from build123d import *

# Parameters (mm, degrees)
SKETCH1_W           = 7.874
SKETCH1_H           = 14.0081
BOSS_EXTRUDE1_DEPTH = 2.54
SKETCH2_W           = 1.101725
SKETCH2_H           = 1.0033
CUT_EXTRUDE1_DEPTH  = 8.636
BOSS_EXTRUDE3_DEPTH = 0.7239


with BuildPart() as part:
    # Sketch1 → Boss-Extrude1 (new body)
    with BuildSketch(Plane(origin=(0, 0, 0), x_dir=(1, 0, 0), z_dir=(0, 1, 0))):
        with Locations((3.937, 7.00405)):
            Rectangle(SKETCH1_W, SKETCH1_H)
    extrude(amount=BOSS_EXTRUDE1_DEPTH)

    # Sketch2 → Cut-Extrude1 (cut)
    with BuildSketch(Plane(origin=(0, 0, -14.0081), x_dir=(-1, 0, 0), z_dir=(0, 0, -1))):
        with Locations((-6.4976375, 1.36525)):
            Rectangle(SKETCH2_W, SKETCH2_H)
        with Locations((-3.971925, 1.36525)):
            Rectangle(SKETCH2_W, SKETCH2_H)
        with Locations((-1.4462125, 1.36525)):
            Rectangle(SKETCH2_W, SKETCH2_H)
    extrude(amount=-CUT_EXTRUDE1_DEPTH, mode=Mode.SUBTRACT)

    # Sketch5 → Boss-Extrude3 (add)
    with BuildSketch(Plane.XZ):
        Polygon((7.874, -14.0081), (7.874, 0), (8.7503, 0), (8.7503, -12.6111), align=None)
    extrude(amount=-BOSS_EXTRUDE3_DEPTH)


solid = part.part
The listing builds one solid part. Answer for the finished solid, in the listing's coordinates (mm). A direction names the side the tool comes from. Coordinates: 2 decimals unless noted, no trailing zeros. Write each loop counter-clockwise with the first axis right and the second up, starting at its lowest first coordinate (ties: lowest second). Pieces come first, ordered by that corner, then holes. Notation, with made-up numbers: M -26.75,66 L -18.75,66 A20 cw -18.75,84 Z; hole C 19.5,10 d9. An arc over 180 degrees is marked long. Write each question's results on one line, items separated by ' | '.
Item 1: Consider probe 1 along Y at (x, z) = (4, -6); probe 2 along X at (y, z) = (1.25, -9); probe 3 along X at (y, z) = (1.1, -4.25). Determine where each line is inside the solid, lowest interval first. Write a range as [from, to].
Answer below:
probe 1: [0, 0.86], [1.87, 2.54] | probe 2: [0, 0.9], [2, 3.42], [4.52, 5.95], [7.05, 7.87] | probe 3: [0, 7.87]
Item 2: The part is cut by section D-D on z = -2.25. Determine the outline of the cut face in (x, y), and give its area (3 significant figures).
Answer below:
outline: M 0,0 L 8.75,0 L 8.75,0.72 L 7.87,0.72 L 7.87,2.54 L 0,2.54 Z | area: 20.6 mm2
Item 3: The part is cut by section B-B on x = 6.5. Determine the outline of the cut face in (y, z), and give its area (3 significant figures).
Answer below:
outline: M 0,-14.01 L 0.86,-14.01 L 0.86,-5.37 L 1.87,-5.37 L 1.87,-14.01 L 2.54,-14.01 L 2.54,0 L 0,0 Z | area: 26.9 mm2
Item 4: Given P1, Ø1.5, axis at y = 2, z = -5, coming from the +X side; P2, Ø0.7, axis at x = 8.5, z = -6, coming from the +Y side, each flat-ended and moving along its own axis, determine where each tip first touches the part or whether it passes through.
Answer below:
P1: x = 7.87 | P2: y = 0.72
Item 5: The part is cut by section C-C on y = 1.35. Determine the outline of the cut face in (x, z), and give its area (3 significant figures).
Answer below:
outline: M 0,-14.01 L 0.9,-14.01 L 0.9,-5.37 L 2,-5.37 L 2,-14.01 L 3.42,-14.01 L 3.42,-5.37 L 4.52,-5.37 L 4.52,-14.01 L 5.95,-14.01 L 5.95,-5.37 L 7.05,-5.37 L 7.05,-14.01 L 7.87,-14.01 L 7.87,0 L 0,0 Z | area: 81.8 mm2
Item 6: Which of the six approach directions +Z, -Z, +X, -X, +Y, -Y give full straight-line access (tool end or side, diameter ignored) to faces 5 (the face through (8.3, 0.724, -6.9)), 6 (the face through (4, 1, 0)), 7 (the face through (6.5, 0.864, -9.8))?
Answer below:
face 5: +Z, -Z, +X, +Y | face 6: +Z, +X, -X, +Y, -Y | face 7: -Z
Item 7: The part is cut by section A-A on z = -10.75. Determine the outline of the cut face in (x, y), and give its area (3 significant figures).
Answer below:
outline: M 0,0 L 8.75,0 L 8.75,0.72 L 7.87,0.72 L 7.87,2.54 L 0,2.54 Z; hole M 0.9,0.86 L 2,0.86 L 2,1.87 L 0.9,1.87 Z; hole M 3.42,0.86 L 4.52,0.86 L 4.52,1.87 L 3.42,1.87 Z; hole M 5.95,0.86 L 7.05,0.86 L 7.05,1.87 L 5.95,1.87 Z | area: 17.3 mm2
Item 8: For a pull along X with two mould halves and no side action, classify faces 1 (the face through (0, 1, -7)), 2 (the face through (8.32, 0.36, -13.3)), 3 (the face through (1.5, 1.4, -5.372)), 4 (the face through (4, 0, -7)) as released by +X, released by -X, zero draft, split by the parting line, or undercut.
Answer below:
face 1: released by -X | face 2: released by +X | face 3: undercut | face 4: zero draft
